Design review of the part built by this model. Coordinates are the model's own, in mm. Face numbers are marked on the shaded views. A direction names the side the tool comes from. Coordinates: 2 decimals unless noted, no trailing zeros. Loops run counter-clockwise (first coordinate to the right, second up) from the corner with the lowest first, then second, coordinate; pieces in that order, holes last. Notation, with made-up numbers: M 87.5,27.5 L 121.5,27.5 A23 ccw 121.5,64.5 Z; hole C 78.5,-9.75 d3. An arc over 180 degrees is marked long. Put each result on its own line as item: value. Start each with the question number.
(1) For probe 1 along X at (y, z) = (9.25, -3); probe 2 along Z at (x, y) = (22, 2.5); probe 3 along X at (y, z) = (6.75, -25.5), list the stretches that pass through material, from the lowest coordinate up. Write a range as [from, to].
(2) Take a section at C-C, the plane x = -13.5. Give the boundary of the cut face in (y, z).
(3) For the marked faces 4, 5 and 6, list the 3-axis set-ups (+Z, -Z, +X, -X, +Y, -Y) from which the entire face can be reached by the end or side of a thin tool; tool diameter is ignored.
(4) Take a section at B-B, the plane z = -22.5. Give the boundary of the cut face in (x, y), then the cut area to 3 significant figures.
(5) The part is to be moulded in two halves that separate along X. For the marked faces 1, 2 and 3, say which applies: +X half, -X half, draft (parallel to the pull), parting line (faces both ways), or undercut.
(6) Clearance check with flat-ended pins moving along their axes: pin 1 (5 mm diameter, centred on x = -4.5, z = 26, fed in from -Y); pin 2 (5 mm diameter, centred on x = 21.87, z = -0.93, fed in from -Y); pin 3 (6 mm diameter, centred on y = 6.5, z = -15, fed in from -X); pin 4 (5 mm diameter, centred on x = -37.5, y = 3.5, fed in from -Z). State where each tip first meets the part, or that it passes through.
(7) Take a section at A-A, the plane y = 1.5. Count the separate pieces of the cut face and the enclosed holes in it, then the cut area to 3 significant figures.
Autodesk Inventor part; units mm, degrees
ref_plane "YZ Plane" through (0, 0, 0) normal (1, 0, 0) x (0, 1, 0)
ref_plane "XZ Plane" through (0, 0, 0) normal (0, 1, 0) x (-1, 0, 0)
ref_plane "XY Plane" through (0, 0, 0) normal (0, 0, 1) x (1, 0, 0)
sketch "Sketch1" plane through (0, 0, 0) normal (0, 1, 0) x (-1, 0, 0)
  circle A0 centre (28.1298, -0.9274) radius 1.5
  circle A1 centre (3.1298, -25.9274) radius 1.5
  circle A2 centre (-21.8702, -0.9274) radius 1.5
  circle A3 centre (3.1298, 24.0726) radius 1.5
  line L0 (33.1298, -30.9274) -> (-26.8702, -30.9274)
  line L1 (-26.8702, -30.9274) -> (-26.8702, 29.0726)
  line L2 (-26.8702, 29.0726) -> (33.1298, 29.0726)
  line L3 (33.1298, 29.0726) -> (33.1298, -30.9274)
  line L4 (33.1298, -30.9274) -> (-26.8702, 29.0726) construction
  line L5 (-26.8702, -30.9274) -> (33.1298, 29.0726) construction
  point P0 (0, 0)
  dimension "d1" = 3
  dimension "d2" = 3
  dimension "d3" = 3
  dimension "d4" = 3
  dimension "d7" = 60
  dimension "d8" = 5
  dimension "d9" = 50
  dimension "d10" = 50
  dimension "d12" = 5
  dimension "d13" = 60
  dimension "d14" = 5
  dimension "d15" = 30
  dimension "d16" = 30
  dimension "d17" = 30
extrude "Extrusion1" add sketch "Sketch1" along normal blind 10
sketch "Sketch2" plane through (0, 10, 0) normal (0, 1, 0) x (1, 0, 0)
  line L0 (26.8702, 30.9274) -> (-33.1298, 30.9274)
  line L1 (-7.7791, 30.9274) -> (2.2209, 30.9274)
  line L2 (2.2209, 30.9274) -> (2.2209, 40.9274)
  line L3 (2.2209, 40.9274) -> (-7.7791, 40.9274)
  line L4 (-7.7791, 40.9274) -> (-7.7791, 30.9274)
  line L5 (-33.1298, -29.0726) -> (26.8702, -29.0726)
  line L6 (-7.7791, -29.0726) -> (2.2209, -29.0726)
  line L7 (2.2209, -29.0726) -> (2.2209, -39.0726)
  line L8 (2.2209, -39.0726) -> (-7.7791, -39.0726)
  line L9 (-7.7791, -39.0726) -> (-7.7791, -29.0726)
  point P0 (0, 0)
  dimension "d18" = 10
  dimension "d19" = 10
  dimension "d20" = 10
extrude "Extrusion2" add sketch "Sketch2" against normal blind 10
sketch "Sketch3" plane through (0, 10, 0) normal (0, 1, 0) x (1, 0, 0)
  circle A0 centre (-2.7791, 36.9274) radius 2.925
  circle A1 centre (-2.7791, -35.0726) radius 2.925
  line L0 (2.2209, 40.9274) -> (-7.7791, 40.9274)
  line L1 (2.2209, -39.0726) -> (-7.7791, -39.0726)
  line L2 (-7.7791, 30.9274) -> (-7.7791, 40.9274)
  line L3 (-7.7791, -39.0726) -> (-7.7791, -29.0726)
  point P0 (0, 0)
  dimension "d23" = 5.85
  dimension "d24" = 5.85
  dimension "d25" = 4
  dimension "d26" = 4
  dimension "d29" = 5
  dimension "d30" = 5
extrude "Extrusion3" cut sketch "Sketch3" against normal through all
sketch "Sketch4" plane through (0, 0, 0) normal (0, -1, 0) x (1, 0, 0)
  circle A0 centre (-3.1298, 24.0726) radius 1.5
  circle A1 centre (-3.1298, 24.0726) radius 4.75
  circle A2 centre (21.8702, -0.9274) radius 1.5
  circle A3 centre (21.8702, -0.9274) radius 4.75
  circle A4 centre (-3.1298, -25.9274) radius 1.5
  circle A5 centre (-3.1298, -25.9274) radius 4.75
  circle A6 centre (-28.1298, -0.9274) radius 1.5
  circle A7 centre (-28.1298, -0.9274) radius 4.75
  point P0 (0, 0)
  dimension "d31" = 9.5
  dimension "d32" = 9.5
  dimension "d33" = 9.5
  dimension "d34" = 9.5
extrude "Extrusion4" cut sketch "Sketch4" against normal blind 7
sketch "Sketch5" plane through (0, 0, 0) normal (0, -1, 0) x (1, 0, 0)
  line L0 (-33.1298, 29.0726) -> (-33.1298, -30.9274)
  line L1 (-33.1298, -5.9274) -> (-43.1298, -5.9274)
  line L2 (-43.1298, -5.9274) -> (-43.1298, 4.0726)
  line L3 (-43.1298, 4.0726) -> (-33.1298, 4.0726)
  line L4 (-33.1298, 4.0726) -> (-33.1298, -5.9274)
  line L5 (-33.1298, -30.9274) -> (-7.7791, -30.9274)
  line L6 (26.8702, 29.0726) -> (-33.1298, 29.0726)
  line L7 (26.8702, -30.9274) -> (26.8702, 29.0726)
  line L8 (26.8702, -5.9274) -> (36.8702, -5.9274)
  line L9 (36.8702, -5.9274) -> (36.8702, 4.0726)
  line L10 (36.8702, 4.0726) -> (26.8702, 4.0726)
  line L11 (26.8702, 4.0726) -> (26.8702, -5.9274)
  line L12 (-33.1298, -30.9274) -> (26.8702, -30.9274)
  line L13 (26.8702, 29.0726) -> (2.2209, 29.0726)
  point P0 (0, 0)
  point P1 (-7.7791, 29.0726)
  point P2 (2.2209, -30.9274)
  dimension "d37" = 10
  dimension "d38" = 10
  dimension "d39" = 25
  dimension "d40" = 25
  dimension "d41" = 10
  dimension "d42" = 25
  dimension "d43" = 25
extrude "Extrusion5" add sketch "Sketch5" against normal blind 10 contours L0 L1 L2 L3 | L10 L9 L8 L7
sketch "Sketch6" plane through (0, 0, 0) normal (0, -1, 0) x (1, 0, 0)
  circle A0 centre (-39.1298, -0.9274) radius 2.925
  circle A1 centre (32.8702, -0.9274) radius 2.925
  line L0 (26.8702, -5.9274) -> (36.8702, -5.9274)
  line L1 (36.8702, -5.9274) -> (36.8702, 4.0726)
  line L2 (-43.1298, -5.9274) -> (-43.1298, 4.0726)
  line L3 (-33.1298, -5.9274) -> (-43.1298, -5.9274)
  point P0 (0, 0)
  dimension "d46" = 5.85
  dimension "d47" = 5.85
  dimension "d48" = 5
  dimension "d49" = 4
  dimension "d50" = 4
  dimension "d51" = 5
extrude "Extrusion6" cut sketch "Sketch6" against normal through all
properties part number "Bottom CLPCLampcell_V5"
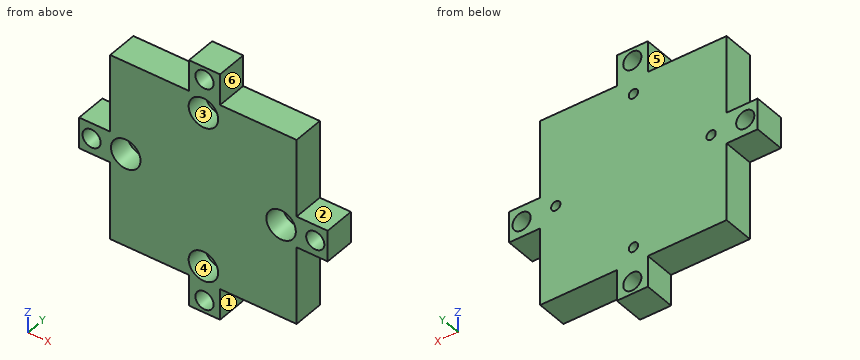
Computed values:
1. probe 1: x = [-43.13, -41.19], [-37.07, 30.81], [34.93, 36.87]
1. probe 2: z = [-30.93, -5.68], [3.82, 29.07]
1. probe 3: x = [-33.13, -7.86], [1.6, 26.87]
2. outline: M 0,-30.93 L 10,-30.93 L 10,29.07 L 0,29.07 Z
3. face 4: -Y
3. face 5: +Z, -X, +Y, -Y
3. face 6: +Z, +X, +Y, -Y
4. outline: M -33.13,0 L -6.42,0 L -6.42,7 L 0.16,7 L 0.16,0 L 26.87,0 L 26.87,10 L -33.13,10 Z
4. area: 554 mm^2
5. face 1: +X half
5. face 2: draft
5. face 3: undercut
6. pin 1: stops at y = 0
6. pin 2: stops at y = 7
6. pin 3: stops at x = -33.13
6. pin 4: stops at z = -5.93
7. separate pieces: 1
7. enclosed holes: 8
7. area: 3,610 mm^2
